Read the model definition and answer for the solid it produces. Units are mm, in the model's axes. A direction names the side the tool comes from. Give positions to 0.01 mm unless a question says otherwise; leave off trailing zeros. Loops run counter-clockwise (first coordinate to the right, second up) from the corner with the lowest first, then second, coordinate; pieces in that order, holes last. Notation, with made-up numbers: (64.5, -19) -> (99.5, -19) arc R9 cw to (99.5, -4) -> close; hole circle Ø11 at (-32.75, -13.75). An arc over 180 degrees is marked (long way). Write each question's results on one line, items separated by ' | '. Start each with the question number.
Item 1: Which of the six approach directions +Z, -Z, +X, -X, +Y, -Y give full straight-line access (tool end or side, diameter ignored) to faces 1 (the flat face through (27, 6.5, 0)), 2 (the flat face through (2, 4, -17.5)), 3 (the flat face through (27, 1.5, 0))?
Item 2: Section B-B on z = 21 is taken. Write down the section's boundary in (x, y), and give its area (3 significant figures).
Item 3: Section A-A on x = 21 is taken. Write down the section's boundary in (y, z).
Item 4: Section C-C on x = 7.5 is taken. Write down the section's boundary in (y, z).
Item 5: Find the intervals of material crossed by line 1 (X direction, y = 3.75, z = 21); line 2 (X direction, y = 7, z = 15); line 3 (Z direction, x = -7, y = 5.75), in increasing order.
Item 6: Section D-D on z = 2 is taken. Write down the section's boundary in (x, y), and give its area (3 significant figures).
Item 7: Each of these flat-tipped pins is pushed along its axis until it touches: P1, Ø3, axis at y = 4, z = 27.5, coming from the +X side; P2, Ø1.5, axis at x = 1.5, y = 4, coming from the -Z side; P3, Ø4.5, axis at y = 3, z = 27.5, coming from the -X side; P4, Ø2.5, axis at x = 21, z = -21, coming from the -Y side. Where does it stop, or does it pass through?
Item 8: Determine the mould class of faces 4 (the flat face through (-18.528, 3.944, -21.573)), 5 (the flat face through (-23, 6.5, 0)), 6 (the flat face through (0, 1.5, 27)) for opening direction Y: +Y half, -Y half, draft (parallel to the pull), parting line (faces both ways), or undercut.
```python
from build123d import *

# Parameters (mm, degrees)
SKETCH1_W         = 50
SKETCH1_H         = 50
SKETCH1_R         = 1.5
SUPPORT_DEPTH     = 8
NORTH_START       = -25
SKETCH2_W         = 20
SKETCH2_H         = 5
NORTH_CUT_DEPTH   = 4
SOUTH_START       = 25
SKETCH2_2_W       = 20
SKETCH2_2_H       = 5
SOUTH_DOWEL_DEPTH = 4
EAST_START        = 25
SKETCH3_W         = 20
SKETCH3_H         = 5
EAST_DOWEL_DEPTH  = 4
WEST_START        = -25
SKETCH3_3_W       = 20
SKETCH3_3_H       = 5
WEST_CUT_DEPTH    = 4


with BuildPart() as part:
    # Sketch1 → Support (new body)
    with BuildSketch(Plane(origin=(0, 0, 0), x_dir=(1, 0, 0), z_dir=(0, 1, 0))):
        Rectangle(SKETCH1_W, SKETCH1_H)
        with Locations(Location((-21, -21, 0), (0, 0, 270))):
            Circle(SKETCH1_R, mode=Mode.SUBTRACT)
        with Locations(Location((21, -21, 0), (0, 0, 270))):
            Circle(SKETCH1_R, mode=Mode.SUBTRACT)
        with BuildLine():
            Line((-13.031373033, 17.5), (17.5, 17.5))
            Line((17.5, 17.5), (17.5, -17.5))
            Line((17.5, -17.5), (-17.5, -17.5))
            Line((-17.5, -17.5), (-17.5, 13.031373033))
            ThreePointArc((-17.5, 13.031373033), (-20, 14.354248689), (-21, 17))
            Line((-21, 17), (-22.130136986, 20.01369863))
            ThreePointArc((-22.130136986, 20.01369863), (-22.060660172, 22.060660172), (-20.01369863, 22.130136986))
            Line((-20.01369863, 22.130136986), (-17, 21))
            ThreePointArc((-17, 21), (-14.354248689, 20), (-13.031373033, 17.5))
        make_face(mode=Mode.SUBTRACT)
        with Locations(Location((21, 21, 0), (0, 0, 270))):
            Circle(SKETCH1_R, mode=Mode.SUBTRACT)
    extrude(amount=SUPPORT_DEPTH)

    # Sketch2 → North Cut (cut)
    with BuildSketch(Plane.XY.offset(NORTH_START)):
        with Locations((0, 4)):
            Rectangle(SKETCH2_W, SKETCH2_H)
    extrude(amount=NORTH_CUT_DEPTH, mode=Mode.SUBTRACT)

    # Sketch2<2> → South Dowel (add)
    with BuildSketch(Plane.XY.offset(SOUTH_START)):
        with Locations((0, 4)):
            Rectangle(SKETCH2_2_W, SKETCH2_2_H)
    extrude(amount=SOUTH_DOWEL_DEPTH)

    # Sketch3 → East Dowel (add)
    with BuildSketch(Plane(origin=(0, 0, 0), x_dir=(0, 0, -1), z_dir=(1, 0, 0)).offset(EAST_START)):
        with Locations((0, 4)):
            Rectangle(SKETCH3_W, SKETCH3_H)
    extrude(amount=EAST_DOWEL_DEPTH)

    # Sketch3<3> → West Cut (cut)
    with BuildSketch(Plane(origin=(0, 0, 0), x_dir=(0, 0, -1), z_dir=(1, 0, 0)).offset(WEST_START)):
        with Locations((0, 4)):
            Rectangle(SKETCH3_3_W, SKETCH3_3_H)
    extrude(amount=WEST_CUT_DEPTH, mode=Mode.SUBTRACT)


solid = part.part
```
Findings:
1) face 1: +Z, -Z, +X, +Y | face 2: +Y, -Y | face 3: +Z, -Z, +X, -Y
2) outline: (-25, 0) -> (-22.5, 0) -> (-22.5, 8) -> (-25, 8) -> close; (-19.5, 0) -> (19.5, 0) -> (19.5, 8) -> (-19.5, 8) -> close; (22.5, 0) -> (25, 0) -> (25, 8) -> (22.5, 8) -> close | area: 352 mm2
3) outline: (0, -25) -> (8, -25) -> (8, -22.5) -> (0, -22.5) -> close; (0, -19.5) -> (8, -19.5) -> (8, 19.5) -> (0, 19.5) -> close; (0, 22.5) -> (8, 22.5) -> (8, 25) -> (0, 25) -> close
4) outline: (0, -25) -> (1.5, -25) -> (1.5, -21) -> (6.5, -21) -> (6.5, -25) -> (8, -25) -> (8, -17.5) -> (0, -17.5) -> close; (0, 17.5) -> (8, 17.5) -> (8, 25) -> (6.5, 25) -> (6.5, 29) -> (1.5, 29) -> (1.5, 25) -> (0, 25) -> close
5) line 1: -25 to -22.5, -19.5 to 19.5, 22.5 to 25 | line 2: -25 to -17.5, 17.5 to 25 | line 3: -21 to -17.5, 17.5 to 29
6) outline: (-25, 0) -> (-17.5, 0) -> (-17.5, 8) -> (-25, 8) -> (-25, 6.5) -> (-21, 6.5) -> (-21, 1.5) -> (-25, 1.5) -> close; (17.5, 0) -> (25, 0) -> (25, 1.5) -> (29, 1.5) -> (29, 6.5) -> (25, 6.5) -> (25, 8) -> (17.5, 8) -> close | area: 120 mm2
7) P1: x = 10 | P2: z = -21 | P3: x = -10 | P4: through
8) face 4: draft | face 5: undercut | face 6: -Y half
